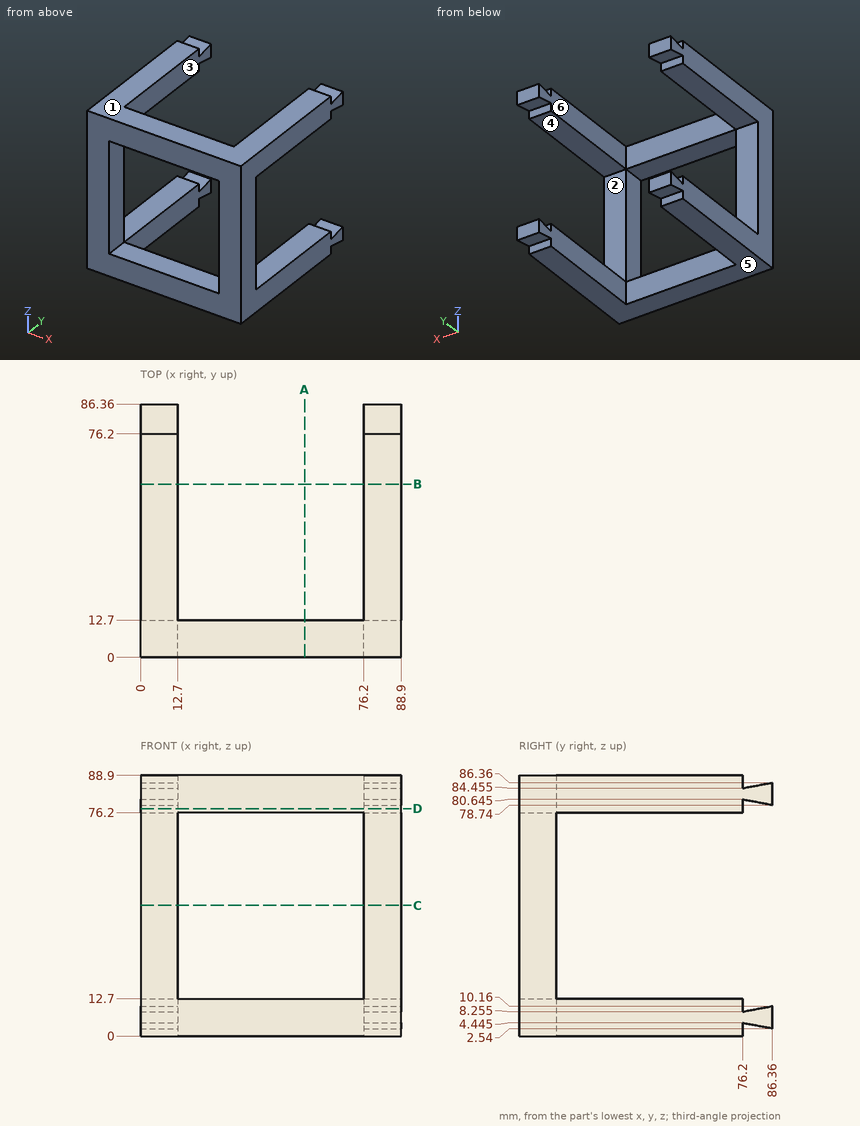
Job drawing, mm, ordinate dimensions from the low corner. One solid piece. A direction names the side the tool comes from. Give positions to 0.01 mm unless a question says otherwise; leave off trailing zeros. Loops run counter-clockwise (first coordinate to the right, second up) from the corner with the lowest first, then second, coordinate; pieces in that order, holes last. Notation, with made-up numbers: M 53,57 L 67,57 A25 ccw 67,94 Z; hole C -33.5,46.25 d4. An arc over 180 degrees is marked long. Answer in a Markdown table with one row per item. Add a question column.
Item 1: Band-saw the part on C-C on z = 44.5. Give the cut face in (x, y).
Item 2: Band-saw the part on A-A on x = 56. Give the cut face in (y, z), then the cut area to 3 significant figures.
Item 3: Band-saw the part on B-B on y = 59. Give the cut face in (x, z).
Item 4: Probe probe 1 along Z at (x, y) = (78.5, 27.5); probe 2 along Y at (x, z) = (4.5, 12.5). List the from-to ranges inside material, lowest first.
Item 5: Band-saw the part on D-D on z = 77.5. Give the cut face in (x, y).
Item 6: Tool access for the marked faces 4, 5 and 6: list every direction of +Z, -Z, +X, -X, +Y, -Y with a clear straight run to the whole face (end or side of a thin tool).
Item 7: Drop flat-ended pins along their axis: P1, Ø10, axis at x = 7, z = 43.5, coming from the +Y side; P2, Ø1.3, axis at x = 8, z = 77.5, coming from the +Y side. Give the stop position or say it passes through.
Item 8: Mould opens along Z. For the marked faces 1, 2 and 3 say: +Z half, -Z half, draft (parallel to the pull), parting line (faces both ways), or undercut.
Reply:
| question | item | result |
|---|---|---|
| 1 | outline | M 0,0 L 12.7,0 L 12.7,12.7 L 0,12.7 Z; M 76.2,0 L 88.9,0 L 88.9,12.7 L 76.2,12.7 Z |
| 2 | outline | M 0,0 L 12.7,0 L 12.7,12.7 L 0,12.7 Z; M 0,76.2 L 12.7,76.2 L 12.7,88.9 L 0,88.9 Z |
| 2 | area | 323 mm^2 |
| 3 | outline | M 0,0 L 12.7,0 L 12.7,12.7 L 0,12.7 Z; M 0,76.2 L 12.7,76.2 L 12.7,88.9 L 0,88.9 Z; M 76.2,0 L 88.9,0 L 88.9,12.7 L 76.2,12.7 Z; M 76.2,76.2 L 88.9,76.2 L 88.9,88.9 L 76.2,88.9 Z |
| 4 | probe 1 | z = 0 to 12.7, 76.2 to 88.9 |
| 4 | probe 2 | y = 0 to 76.2 |
| 5 | outline | M 0,0 L 88.9,0 L 88.9,76.2 L 76.2,76.2 L 76.2,12.7 L 12.7,12.7 L 12.7,76.2 L 0,76.2 Z |
| 6 | face 4 | +X, -X, +Y |
| 6 | face 5 | -Z, +X, -X, +Y, -Y |
| 6 | face 6 | +Z, -Z, +Y |
| 7 | P1 | stops at y = 12.7 |
| 7 | P2 | stops at y = 76.2 |
| 8 | face 1 | +Z half |
| 8 | face 2 | undercut |
| 8 | face 3 | draft |
